from build123d import *

# Parameters (mm, degrees)
SKETCH1_W               = 40
SKETCH1_H               = 42
BOSS_EXTRUDE1_DEPTH     = 3.175
SKETCH2_R               = 1
CUT_EXTRUDE1_DEPTH      = 4.175
SKETCH3_W               = 50.8
SKETCH3_H               = 63.5
BOSS_EXTRUDE2_DEPTH     = 3.175
SKETCH4_R               = 2.032
CUT_EXTRUDE2_DEPTH      = 4.175
SKETCH8_R               = 1.651
CUT_EXTRUDE5_DEPTH      = 4.175
SKETCH9_R               = 15.24
CUT_EXTRUDE6_DEPTH      = 4.175
SKETCH10_W              = 50.8
SKETCH10_H              = 21.5
CUT_EXTRUDE7_DEPTH      = 1
CUT_EXTRUDE7_DEPTH_BACK = 4.175


with BuildPart() as part:
    # Sketch1 → Boss-Extrude1 (new body)
    with BuildSketch(Plane(origin=(0, 0, 0), x_dir=(1, 0, 0), z_dir=(0, 1, 0))):
        Rectangle(SKETCH1_W, SKETCH1_H)
    extrude(amount=BOSS_EXTRUDE1_DEPTH)

    # Sketch2 → Cut-Extrude1 (cut, through all)
    with BuildSketch(Plane(origin=(0, 3.175, 0), x_dir=(1, 0, 0), z_dir=(0, 1, 0))):
        with Locations((17.015999872, -17.952)):
            Circle(SKETCH2_R)
        with Locations((-17.015999872, -17.952)):
            Circle(SKETCH2_R)
        with Locations((17.015999872, 17.952)):
            Circle(SKETCH2_R)
        with Locations((-17.015999872, 17.952)):
            Circle(SKETCH2_R)
    extrude(amount=-CUT_EXTRUDE1_DEPTH, mode=Mode.SUBTRACT)

    # Sketch3 → Boss-Extrude2 (add)
    with BuildSketch(Plane(origin=(0, 3.175, 0), x_dir=(1, 0, 0), z_dir=(0, 1, 0))):
        with Locations((45.4, -10.75)):
            Rectangle(SKETCH3_W, SKETCH3_H)
        with Locations((-45.4, -10.75)):
            Rectangle(SKETCH3_W, SKETCH3_H)
    extrude(amount=-BOSS_EXTRUDE2_DEPTH)

    # Sketch4 → Cut-Extrude2 (cut, through all)
    with BuildSketch(Plane(origin=(0, 3.175, 0), x_dir=(1, 0, 0), z_dir=(0, 1, 0))):
        with Locations((63.18, 8.3)):
            Circle(SKETCH4_R)
        with Locations((37.814543867, 8.3)):
            Circle(SKETCH4_R)
        with Locations((-37.78, 8.3)):
            Circle(SKETCH4_R)
        with Locations((-63.18, 8.3)):
            Circle(SKETCH4_R)
    extrude(amount=-CUT_EXTRUDE2_DEPTH, mode=Mode.SUBTRACT)

    # Sketch8 → Cut-Extrude5 (cut, through all)
    with BuildSketch(Plane(origin=(0, 0, 0), x_dir=(-1, 0, 0), z_dir=(0, -1, 0))):
        with Locations((-32.7, -38.69)):
            Circle(SKETCH8_R)
        with Locations((-32.7, -11.766)):
            Circle(SKETCH8_R)
        with Locations((-59.624, -38.69)):
            Circle(SKETCH8_R)
        with Locations((-59.624, -11.766)):
            Circle(SKETCH8_R)
    extrude(amount=-CUT_EXTRUDE5_DEPTH, mode=Mode.SUBTRACT)

    # Sketch9 → Cut-Extrude6 (cut, through all)
    with BuildSketch(Plane(origin=(0, 0, 0), x_dir=(-1, 0, 0), z_dir=(0, -1, 0))):
        with Locations((-46.162, -25.228)):
            Circle(SKETCH9_R)
    extrude(amount=-CUT_EXTRUDE6_DEPTH, mode=Mode.SUBTRACT)

    # Sketch10 → Cut-Extrude7 (cut, two sides)
    with BuildSketch(Plane(origin=(0, 3.175, 0), x_dir=(1, 0, 0), z_dir=(0, 1, 0))) as cut_extrude7_sk:
        with Locations((-45.4, -31.75)):
            Rectangle(SKETCH10_W, SKETCH10_H)
    extrude(amount=CUT_EXTRUDE7_DEPTH, mode=Mode.SUBTRACT)
    extrude(cut_extrude7_sk.sketch, amount=-CUT_EXTRUDE7_DEPTH_BACK, mode=Mode.SUBTRACT)


solid = part.part
Could you check a few things on this model? Use its own coordinates, in mm. A direction names the side the tool comes from. Round coordinates to 2 decimals unless told otherwise and drop trailing zeros. Order: outer loops, then holes, each group sorted by start corner. A loop starts at its lowest first (then second) coordinate and runs counter-clockwise, first axis right, second up. Notation, with made-up numbers: M 24,-36 L 74,-36 A21 ccw 74,-18 Z; hole C 21,17 d5. An arc over 180 degrees is marked long. One line per item, written item: value.
(1) Imagine slicing it at C-C (y = 2.3). Count the separate pieces of the cut face and the enclosed holes in it, and give its area (3 significant figures).
Ans:
separate pieces: 1
enclosed holes: 13
area: 6,210 mm^2
(2) I need wall thicknesses on line 1 along X through (y, z) = (2.55, -8.3); line 2 along X through (y, z) = (1.45, 38.69) (3 decimals); line 3 along Z through (x, y) = (32.7, 1.6) (3 decimals). Which ranges of each line are inside material? Lowest first, please. Write a range as from..to.
Ans:
line 1: x = -70.8..-65.21, -61.15..-39.81, -35.75..35.78, 39.85..61.15, 65.21..70.8
line 2: x = 20..31.049, 34.351..39.018, 53.306..57.973, 61.275..70.8
line 3: z = -21..10.115, 13.417..18.084, 32.372..37.039, 40.341..42.5
(3) Which directions (+Z, -Z, +X, -X, +Y, -Y) give clear straight access to the entire face, cutting with the end or side of a thin tool? Please do faces 5 (the flat face through (20, 2, 32)), 6 (the flat face through (-1, 0, 3)).
Ans:
face 5: +Z, -X, +Y, -Y
face 6: +Z, -Z, +X, -X, -Y
(4) If we mould it in two halves opening along Z, with no side actions, what happens to faces 1 (the flat face through (-1, 2, -21)), 2 (the flat face through (45, 2, 42.5)), 3 (the cylindrical face through (34.35, 1.57, 11.69)), 4 (the flat face through (-1, 3.175, 3))? For each: released by +Z, released by -Z, zero draft, split by the parting line, or undercut.
Ans:
face 1: released by -Z
face 2: released by +Z
face 3: undercut
face 4: zero draft
(5) I'm going to push flat-ended pins straight in: P1, Ø5.5, axis at x = 63.18, z = -8.3, coming from the -Y side; P2, Ø1.5, axis at x = -44, y = 1, coming from the +Z side; P3, Ø1.2, axis at x = 17.016, z = 17.952, coming from the +Y side; P4, Ø1, axis at y = 2, z = 28.5, coming from the -X side. Where does each tip first touch, or does it pass through?
Ans:
P1: stops at y = 0
P2: stops at z = 21
P3: passes through
P4: stops at x = 20
(6) Imagine slicing it at D-D (x = 32.7). Write out the boundary of the cut face in (y, z) (3 decimals).
Ans:
outline: M 0,-21 L 3.175,-21 L 3.175,10.115 L 0,10.115 Z; M 0,13.417 L 3.175,13.417 L 3.175,18.084 L 0,18.084 Z; M 0,32.372 L 3.175,32.372 L 3.175,37.039 L 0,37.039 Z; M 0,40.341 L 3.175,40.341 L 3.175,42.5 L 0,42.5 Z
(7) Imagine slicing it at A-A (x = 63.18). Write out the boundary of the cut face in (y, z) (3 decimals).
Ans:
outline: M 0,-21 L 3.175,-21 L 3.175,-10.332 L 0,-10.332 Z; M 0,-6.268 L 3.175,-6.268 L 3.175,42.5 L 0,42.5 Z
(8) Imagine slicing it at B-B (z = 38.69). Write out the boundary of the cut face in (x, y) (3 decimals).
Ans:
outline: M 20,0 L 31.049,0 L 31.049,3.175 L 20,3.175 Z; M 34.351,0 L 39.018,0 L 39.018,3.175 L 34.351,3.175 Z; M 53.306,0 L 57.973,0 L 57.973,3.175 L 53.306,3.175 Z; M 61.275,0 L 70.8,0 L 70.8,3.175 L 61.275,3.175 Z
